```python
from build123d import *

# Parameters (mm, degrees)
F0_R     = 1.25
F0_R_2   = 2.75
F1_DEPTH = 8
F2_R     = 5
F3_DEPTH = 4


with BuildPart() as f1:
    # F0 (on Front) → F1 (new body)
    with BuildSketch(Plane.XZ):
        with BuildLine():
            Line((67.5, -15), (67.5, 15))
            Line((67.5, 15), (-62.229646, 15))
            ThreePointArc((-62.229646, 15), (-66.892095, 16.153443), (-70.47897, 19.347686))
            Line((-70.47897, 19.347686), (-89.187697, 46.652314))
            ThreePointArc((-89.187697, 46.652314), (-92.774572, 49.846557), (-97.437021, 51))
            Line((-97.437021, 51), (-156.5, 51))
            Line((-156.5, 51), (-156.5, 39))
            Line((-156.5, 39), (-118.770354, 39))
            ThreePointArc((-118.770354, 39), (-114.107905, 37.846557), (-110.52103, 34.652314))
            Line((-110.52103, 34.652314), (-79.47897, -10.652314))
            ThreePointArc((-79.47897, -10.652314), (-75.892095, -13.846557), (-71.229646, -15))
            Line((-71.229646, -15), (67.5, -15))
        make_face()
        with Locations((52.5, -11)):
            Circle(F0_R, mode=Mode.SUBTRACT)
        with Locations((52.5, 11)):
            Circle(F0_R, mode=Mode.SUBTRACT)
        with Locations((-150.25, 45)):
            Circle(F0_R_2, mode=Mode.SUBTRACT)
        with Locations((-133.25, 45)):
            Circle(F0_R_2, mode=Mode.SUBTRACT)
    extrude(amount=F1_DEPTH)

    # F2 (on face) → F3 (cut)
    with BuildSketch(Plane.XZ.offset(8)):
        with Locations((-150.25, 45)):
            Circle(F2_R)
        with Locations((-133.25, 45)):
            Circle(F2_R)
    extrude(amount=-F3_DEPTH, mode=Mode.SUBTRACT)


solid = f1.part
```
Part model, mm, in its own coordinate system. A direction names the side the tool comes from. Round coordinates to 2 decimals unless told otherwise and drop trailing zeros. Write each loop counter-clockwise with the first axis right and the second up, starting at its lowest first coordinate (ties: lowest second). Pieces come first, ordered by that corner, then holes. Notation, with made-up numbers: M 78,9.5 L 103,9.5 A27 cw 103,31.5 Z; hole C 18,-21 d3. An arc over 180 degrees is marked long. Answer as CSV lines item,"result". Start each with the question number.
1) Band-saw the part on A-A (x = -133.25). List the corners of the cut face in (y, z).
2) Drill centre lines: L1, parallel to Z at x = 52.5, y = -2.5; L2, parallel to Z at x = -150.25, y = -2.2; L3, parallel to X at y = -1, z = 44.5. Where is each one in solid material? Low to high.
3) Band-saw the part on B-B (y = -1.25). List the corners of the cut face in (x, z).
4) Band-saw the part on C-C (x = -40.5). List the corners of the cut face in (y, z).
5) Mould opens along Z. For faces 1 (the face through (-131, -4, 43)), 2 (the face through (-66.83, -3.94, 16.12)), 3 (the face through (-46, 0, 11)) say: +Z half, -Z half, draft (parallel to the pull), parting line (faces both ways), or undercut.
6) Which spindle directions (+Z, -Z, +X, -X, +Y, -Y) get a long thin tool onto all of the face, cutting with end or side? Do faces 4 (the face through (-147.63, -1.97, 45.83)), 5 (the face through (-138, -4, 39)), 6 (the face through (-130.562, -6.028, 49.216)). Say none if no direction does.
7) Band-saw the part on D-D (z = 30.5). List the corners of the cut face in (x, y), then the cut area to 3 significant figures.
8) Drop flat-ended pins along their axis: pin 1 (2.5 mm diameter, centred on x = -128.5, y = -3.5, fed in from -Z); pin 2 (3 mm diameter, centred on x = -131, z = 44, fed in from -Y). Give the stop position or say it passes through.
Worked out:
1,outline,"M -8,39 L 0,39 L 0,42.25 L -4,42.25 L -4,40 L -8,40 Z; M -8,50 L -4,50 L -4,47.75 L 0,47.75 L 0,51 L -8,51 Z"
2,L1,"-15 to -12.25, -9.75 to 9.75, 12.25 to 15"
2,L2,"39 to 42.25, 47.75 to 51"
2,L3,"-156.5 to -152.95, -147.55 to -135.95, -130.55 to -87.71"
3,outline,"M -156.5,39 L -118.77,39 A10 cw -110.52,34.65 L -79.48,-10.65 A10 ccw -71.23,-15 L 67.5,-15 L 67.5,15 L -62.23,15 A10 cw -70.48,19.35 L -89.19,46.65 A10 ccw -97.44,51 L -156.5,51 Z; hole C -150.25,45 d5.5; hole C -133.25,45 d5.5; hole C 52.5,-11 d2.5; hole C 52.5,11 d2.5"
4,outline,"M -8,-15 L 0,-15 L 0,15 L -8,15 Z"
5,face 1,"undercut"
5,face 2,"+Z half"
5,face 3,"draft"
6,face 4,"+Y, -Y"
6,face 5,"-Z, -X, +Y, -Y"
6,face 6,"-Y"
7,outline,"M -107.68,-8 L -78.12,-8 L -78.12,0 L -107.68,0 Z"
7,area,"236 mm²"
8,pin 1,"z = 39"
8,pin 2,"y = -4"
